Geometry: final body of the model. Coordinates: model frame, mm. A direction names the side the tool comes from. Round coordinates to 2 decimals unless told otherwise and drop trailing zeros. Write each loop counter-clockwise with the first axis right and the second up, starting at its lowest first coordinate (ties: lowest second). Pieces come first, ordered by that corner, then holes.
from build123d import *

# Parameters (mm, degrees)
SKETCH1_W               = 44
SKETCH1_H               = 63.5
SKETCH1_W_2             = 38.55
SKETCH1_H_2             = 12.661180653
BOSS_EXTRUDE1_DEPTH     = 19.038019
SKETCH1_3_W             = 38.55
SKETCH1_3_H             = 12.661180653
BOSS_EXTRUDE2_DEPTH     = 19.061980653
CUT_EXTRUDE1_DEPTH      = 197.962748017
CUT_EXTRUDE1_DEPTH_BACK = 197.962748017
SKETCH2_R               = 3.96875
CUT_EXTRUDE2_START      = -31.75
SKETCH2_3_R             = 8.89
SKETCH2_3_R_2           = 3.96875
CUT_EXTRUDE2_DEPTH      = 7.103661
CUT_EXTRUDE3_START      = 24.646339347
SKETCH2_4_R             = 8.89
SKETCH2_4_R_2           = 3.96875
CUT_EXTRUDE3_DEPTH      = 7.103660653
SKETCH3_R               = 2.65
CUT_EXTRUDE4_DEPTH      = 197.962748017
CUT_EXTRUDE5_START      = 6.349999653
SKETCH3_3_R             = 4.75
SKETCH3_3_R_2           = 2.65
SKETCH3_3_R_3           = 2.5
CUT_EXTRUDE5_DEPTH      = 12.688019347


with BuildPart() as part:
    # Sketch1 → Boss-Extrude1 (new body)
    with BuildSketch(Plane.XY):
        with Locations((-171.45, 0)):
            Rectangle(SKETCH1_W, SKETCH1_H)
        with Locations((-130.175, -25.419409674)):
            Rectangle(SKETCH1_W_2, SKETCH1_H_2)
        with Locations((-130.175, 25.419409674)):
            Rectangle(SKETCH1_W_2, SKETCH1_H_2)
    extrude(amount=BOSS_EXTRUDE1_DEPTH)

    # Sketch1<3> → Boss-Extrude2 (add)
    with BuildSketch(Plane.XY):
        with Locations((-130.175, 25.419409674)):
            Rectangle(SKETCH1_3_W, SKETCH1_3_H)
        with Locations((-130.175, -25.419409674)):
            Rectangle(SKETCH1_3_W, SKETCH1_3_H)
    extrude(amount=-BOSS_EXTRUDE2_DEPTH)

    # Sketch2 → Cut-Extrude1 (cut, two sides: drawn at the far end of the back side and taken through both)
    with BuildSketch(Plane(origin=(0, 0, 0), x_dir=(1, 0, 0), z_dir=(0, 1, 0)).offset(-CUT_EXTRUDE1_DEPTH_BACK)):
        with Locations(Location((-130.175, 0.011980653, 0), (0, 0, 270))):
            Circle(SKETCH2_R)
    extrude(amount=CUT_EXTRUDE1_DEPTH + CUT_EXTRUDE1_DEPTH_BACK, mode=Mode.SUBTRACT)

    # Sketch2<3> → Cut-Extrude2 (cut)
    with BuildSketch(Plane(origin=(0, 0, 0), x_dir=(1, 0, 0), z_dir=(0, 1, 0)).offset(CUT_EXTRUDE2_START)):
        with Locations(Location((-130.175, 0.011980653, 0), (0, 0, 270))):
            Circle(SKETCH2_3_R)
        with Locations(Location((-130.175, 0.011980653, 0), (0, 0, 270))):
            Circle(SKETCH2_3_R_2, mode=Mode.SUBTRACT)
    extrude(amount=CUT_EXTRUDE2_DEPTH, mode=Mode.SUBTRACT)

    # Sketch2<4> → Cut-Extrude3 (cut)
    with BuildSketch(Plane(origin=(0, 0, 0), x_dir=(1, 0, 0), z_dir=(0, 1, 0)).offset(CUT_EXTRUDE3_START)):
        with Locations(Location((-130.175, 0.011980653, 0), (0, 0, 270))):
            Circle(SKETCH2_4_R)
        with Locations(Location((-130.175, 0.011980653, 0), (0, 0, 270))):
            Circle(SKETCH2_4_R_2, mode=Mode.SUBTRACT)
    extrude(amount=CUT_EXTRUDE3_DEPTH, mode=Mode.SUBTRACT)

    # Sketch3 → Cut-Extrude4 (cut, through all)
    with BuildSketch(Plane.XY):
        with Locations((-187.45, 18)):
            Circle(SKETCH3_R)
        with Locations((-155.45, 18)):
            Circle(SKETCH3_R)
        with Locations((-155.45, -18)):
            Circle(SKETCH3_R)
        with Locations((-187.45, -18)):
            Circle(SKETCH3_R)
    extrude(amount=CUT_EXTRUDE4_DEPTH, mode=Mode.SUBTRACT)

    # Sketch3<3> → Cut-Extrude5 (cut)
    # profile 1 of 8: a face of its own
    with BuildSketch(Plane.XY.offset(CUT_EXTRUDE5_START)):
        with Locations((-187.45, 18)):
            Circle(SKETCH3_3_R)
        with Locations((-187.45, 18)):
            Circle(SKETCH3_3_R_2, mode=Mode.SUBTRACT)
    # profile 2 of 8: a face of its own
    with BuildSketch(Plane.XY.offset(CUT_EXTRUDE5_START)):
        with Locations((-187.45, 18)):
            Circle(SKETCH3_3_R_3)
    # profile 3 of 8: a face of its own
    with BuildSketch(Plane.XY.offset(CUT_EXTRUDE5_START)):
        with Locations((-155.45, 18)):
            Circle(SKETCH3_3_R)
        with Locations((-155.45, 18)):
            Circle(SKETCH3_3_R_2, mode=Mode.SUBTRACT)
    # profile 4 of 8: a face of its own
    with BuildSketch(Plane.XY.offset(CUT_EXTRUDE5_START)):
        with Locations((-155.45, 18)):
            Circle(SKETCH3_3_R_3)
    # profile 5 of 8: a face of its own
    with BuildSketch(Plane.XY.offset(CUT_EXTRUDE5_START)):
        with Locations((-155.45, -18)):
            Circle(SKETCH3_3_R)
        with Locations((-155.45, -18)):
            Circle(SKETCH3_3_R_2, mode=Mode.SUBTRACT)
    # profile 6 of 8: a face of its own
    with BuildSketch(Plane.XY.offset(CUT_EXTRUDE5_START)):
        with Locations((-155.45, -18)):
            Circle(SKETCH3_3_R_3)
    # profile 7 of 8: a face of its own
    with BuildSketch(Plane.XY.offset(CUT_EXTRUDE5_START)):
        with Locations((-187.45, -18)):
            Circle(SKETCH3_3_R)
        with Locations((-187.45, -18)):
            Circle(SKETCH3_3_R_2, mode=Mode.SUBTRACT)
    # profile 8 of 8: a face of its own
    with BuildSketch(Plane.XY.offset(CUT_EXTRUDE5_START)):
        with Locations((-187.45, -18)):
            Circle(SKETCH3_3_R_3)
    extrude(amount=CUT_EXTRUDE5_DEPTH, mode=Mode.SUBTRACT)


solid = part.part
1) Section D-D on x = -187.45. Output: boundary loops of the cut face in (y, z).
2) Section B-B on z = -15. Output: boundary loops of the cut face in (x, y).
3) Section C-C on y = -18. Output: boundary loops of the cut face in (x, z).
4) Section A-A on x = -145.5. Output: boundary loops of the cut face in (y, z), plus the area to 3 significant figures.
5) Reachability of faces 1 (the cylindrical face through (-152.922, 18.796, 3.131)), 2 (the flat face through (-130, -19.089, -5)), 3 (the cylindrical face through (-160.195, -17.791, 12.605)), 4 (the flat face through (-132, 24.646, 4)), 5 (the cylindrical face through (-121.36, -28.25, -1.17)) from +Z, -Z, +X, -X, +Y, -Y: full face, straight path, thin tool, end or side. Return the list, or none.
6) Draft query along Y for faces 6 (the flat face through (-153, 31.75, 4)), 7 (the cylindrical face through (-134.05, 21.83, -0.87)), 8 (the cylindrical face through (-160.195, 18.209, 12.605)). Return one class per face: pulls with the +Y half, pulls with the -Y half, needs draft (parallel to the pull), parting line crosses it, or undercut.
7) Line query: probe 1 along Y at (x, z) = (-155.45, 4.5); probe 2 along Y at (x, z) = (-187, 17); probe 3 along Y at (x, z) = (-115.5, -8.5). Output: solid intervals per line, ascending.
8) First-contact query: P1, Ø12.5, axis at x = -130.18, z = -0.01, coming from the +Y side; P2, Ø3, axis at x = -186, y = -18, coming from the +Z side; P3, Ø9.5, axis at y = -1.5, z = 12.5, coming from the +X side. Flat tips, straight axial feed; report the tip coordinate or a pass-through.
Filled in:
1. outline: (-31.75, 0) - (-20.65, 0) - (-20.65, 6.35) - (-22.75, 6.35) - (-22.75, 19.04) - (-31.75, 19.04) - close; (-15.35, 0) - (15.35, 0) - (15.35, 6.35) - (13.25, 6.35) - (13.25, 19.04) - (-13.25, 19.04) - (-13.25, 6.35) - (-15.35, 6.35) - close; (20.65, 0) - (31.75, 0) - (31.75, 19.04) - (22.75, 19.04) - (22.75, 6.35) - (20.65, 6.35) - close
2. outline: (-149.45, -31.75) - (-110.9, -31.75) - (-110.9, -19.09) - (-149.45, -19.09) - close; (-149.45, 19.09) - (-110.9, 19.09) - (-110.9, 31.75) - (-149.45, 31.75) - close
3. outline: (-193.45, 0) - (-190.1, 0) - (-190.1, 6.35) - (-192.2, 6.35) - (-192.2, 19.04) - (-193.45, 19.04) - close; (-184.8, 0) - (-158.1, 0) - (-158.1, 6.35) - (-160.2, 6.35) - (-160.2, 19.04) - (-182.7, 19.04) - (-182.7, 6.35) - (-184.8, 6.35) - close; (-152.8, 0) - (-149.45, 0) - (-149.45, 19.04) - (-150.7, 19.04) - (-150.7, 6.35) - (-152.8, 6.35) - close
4. outline: (-31.75, -19.06) - (-19.09, -19.06) - (-19.09, 19.04) - (-31.75, 19.04) - close; (19.09, -19.06) - (31.75, -19.06) - (31.75, 19.04) - (19.09, 19.04) - close
4. area: 965 mm2
5. face 1: +Z, -Z
5. face 2: +Z, -Z, +X
5. face 3: +Z
5. face 4: +Y
5. face 5: -Y
6. face 6: pulls with the +Y half
6. face 7: needs draft
6. face 8: undercut
7. probe 1: y = -31.75 to -20.65, -15.35 to 15.35, 20.65 to 31.75
7. probe 2: y = -31.75 to -22.73, -13.27 to 13.27, 22.73 to 31.75
7. probe 3: y = -31.75 to -19.09, 19.09 to 31.75
8. P1: stops at y = 24.65
8. P2: stops at z = 6.35
8. P3: stops at x = -149.45
